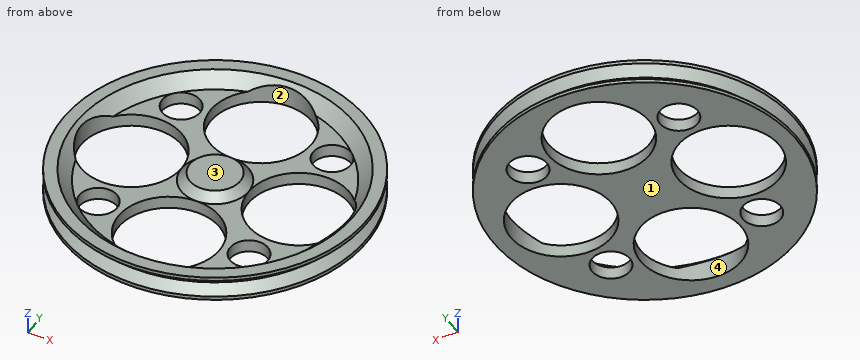
```python
from build123d import *

# Parameters (mm, degrees)
SKETCH001_R           = 12
SKETCH001_R_2         = 4.5
POCKET_DEPTH          = 210.001
POLARPATTERN001_COUNT = 4


with BuildPart() as part:
    # Sketch → Revolution (revolve)
    with BuildSketch(Plane.XZ):
        Polygon((0, 2), (-5.985281, 2), (-8, 0), (-29.955844, 0), (-32.977922, 3), (-36, 3), (-36, 2.12132), (-33.87868, 0), (-36, -2.12132), (-36, -3), (0, -3), align=None)
    revolve(axis=Axis((0, 0, 0), (0, 0, 1)))

    # Sketch001 → Pocket (cut, through all)
    with BuildSketch(Plane(origin=(0, 0, -3), x_dir=(1, 0, 0), z_dir=(0, 0, -1))):
        with Locations((0, 20)):
            Circle(SKETCH001_R)
        with Locations((18, 18)):
            Circle(SKETCH001_R_2)
    pocket = extrude(amount=-POCKET_DEPTH, mode=Mode.SUBTRACT)

    # PolarPattern001: Pocket ×4 about axis
    polarpattern001_axis = Axis((0, 0, -3), (0, 0, -1))
    for i in range(1, POLARPATTERN001_COUNT):
        add(pocket.rotate(polarpattern001_axis, i * 360 / POLARPATTERN001_COUNT), mode=Mode.SUBTRACT)


solid = part.part
```
Can you work these out from the model? Positions are in its coordinate system, mm. Face numbers are marked on the shaded views. A direction names the side the tool comes from. Round coordinates to 2 decimals unless told otherwise and drop trailing zeros. One line per item, written item: value. Start each with the question number.
1. For the marked faces 3 and 4, which set-ups out of +Z, -Z, +X, -X, +Y, -Y let a thin tool reach every point of the face, with its end or its side?
2. For pin 1 (2 mm diameter, centred on x = -4.5, z = -1.5, fed in from +Y); pin 2 (23 mm diameter, centred on x = -18, y = -12, fed in from +Z); pin 3 (3 mm diameter, centred on x = -5.5, z = -0.5, fed in from -Y); pin 4 (3.5 mm diameter, centred on x = 1, y = 2, fed in from +Z), each with a flat end and sliding along its axis, tell me the tip position at first contact or that it passes through.
3. If we section it at A-A, the plane z = -1: Give the number of separate pieces and of enclosed holes in the cut face, then the cut area to 3 significant figures.
4. If we mould it in two halves opening along X, with no side actions, what happens to the marked faces 1 and 2? For each: pulls with the +X half, pulls with the -X half, needs draft (parallel to the pull), parting line crosses it, or undercut.
5. If I drill on probe 1 along Y at (x, z) = (4.5, -0.5); probe 2 along Y at (x, z) = (0, 0.8); probe 3 along X at (y, z) = (-18, -1.5), over which ranges is the centre line in solid material (lowest first)?
Calculated:
1. face 3: +Z
1. face 4: +Z, -Z
2. pin 1: stops at y = 35.81
2. pin 2: stops at z = 3
2. pin 3: stops at y = -35.47
2. pin 4: stops at z = 2
3. separate pieces: 1
3. enclosed holes: 8
3. area: 1,760 mm²
4. face 1: needs draft
4. face 2: undercut
5. probe 1: y = -34.08 to -31.12, -8.88 to 8.88, 31.12 to 34.08
5. probe 2: y = -34.68 to -32, -7.19 to 7.19, 32 to 34.68
5. probe 3: x = -30.46 to -22.5, -13.5 to -11.83, 11.83 to 13.5, 22.5 to 30.46
